```python
from build123d import *
from build123d.topology import SkipClean

# Parameters (mm, degrees)
SKETCH_1_R           = 112.5
SKETCH_1_R_2         = 90
EXTRUDE_1_DEPTH      = 3
EXTRUDE_START        = -60
EXTRUDE_2_DEPTH      = 60
SKETCH_5_R           = 2.75
CUT_EXTRUDE_1_DEPTH  = 10
EXTRUDE_3_DEPTH      = 5
EXTRUDE_3_DEPTH_BACK = 3
SKETCH_6_R           = 115.5
SKETCH_6_R_2         = 112.5
EXTRUDE_START_2      = 10
EXTRUDE_4_DEPTH      = 10


with BuildPart() as part:
    # Sketch 1 → Extrude 1 (new body)
    with BuildSketch(Plane.XY):
        Circle(SKETCH_1_R)
        Circle(SKETCH_1_R_2, mode=Mode.SUBTRACT)
    extrude(amount=EXTRUDE_1_DEPTH)

    # Sketch 4 → Extrude 2 (add)
    with BuildSketch(Plane.XY.offset(3).offset(EXTRUDE_START)):
        with BuildLine():
            Line((-25, 109.687054842), (-25, 112.76191733))
            ThreePointArc((-25, 112.76191733), (0, -115.5), (25, 112.76191733))
            Line((25, 112.76191733), (25, 109.687054842))
            ThreePointArc((25, 109.687054842), (0, -112.5), (-25, 109.687054842))
        make_face()
    extrude(amount=EXTRUDE_2_DEPTH)

    # Sketch 5 → Cut-Extrude 1 (cut)
    with BuildSketch(Plane.XY.offset(3)):
        with Locations((80, 60)):
            Circle(SKETCH_5_R)
        with Locations((92.803208809, 37.250025969)):
            Circle(SKETCH_5_R)
        with Locations((61.744923397, 78.661073186)):
            Circle(SKETCH_5_R)
        with Locations((61.744923397, -78.661073186)):
            Circle(SKETCH_5_R)
        with Locations((92.803208809, -37.250025969)):
            Circle(SKETCH_5_R)
        with Locations((80, -60)):
            Circle(SKETCH_5_R)
        with Locations((-80, -60)):
            Circle(SKETCH_5_R)
        with Locations((-92.803208809, -37.250025969)):
            Circle(SKETCH_5_R)
        with Locations((-61.744923397, -78.661073186)):
            Circle(SKETCH_5_R)
        with Locations((-61.744923397, 78.661073186)):
            Circle(SKETCH_5_R)
        with Locations((-92.803208809, 37.250025969)):
            Circle(SKETCH_5_R)
        with Locations((-80, 60)):
            Circle(SKETCH_5_R)
        with Locations((15, 105)):
            Circle(SKETCH_5_R)
        with Locations((-15, 105)):
            Circle(SKETCH_5_R)
    extrude(amount=-CUT_EXTRUDE_1_DEPTH, mode=Mode.SUBTRACT)

    # Sketch 6 → Extrude 3 (add, two sides: drawn at the far end of the back side and taken through both)
    with SkipClean():  # the faces are left unmerged after this step: merging them gives an invalid solid
        with BuildSketch(Plane(origin=(0, 0, 0), x_dir=(-1, 0, 0), z_dir=(0, 0, -1)).offset(-EXTRUDE_3_DEPTH_BACK)):
            with Locations(Location((0, 0, 0), (0, 0, 180))):
                Circle(SKETCH_6_R)
            with Locations(Location((0, 0, 0), (0, 0, 180))):
                Circle(SKETCH_6_R_2, mode=Mode.SUBTRACT)
        extrude(amount=EXTRUDE_3_DEPTH + EXTRUDE_3_DEPTH_BACK)

    # Sketch 7 → Extrude 4 (add)
    with SkipClean():  # the faces are left unmerged after this step: merging them gives an invalid solid
        with BuildSketch(Plane(origin=(0, 0, -57), x_dir=(-1, 0, 0), z_dir=(0, 0, -1)).offset(EXTRUDE_START_2)):
            with BuildLine():
                Line((-48.117044797, 105), (48.117044797, 105))
                ThreePointArc((48.117044797, 105), (36.763941575, 109.492751358), (25, 112.76191733))
                Line((25, 112.76191733), (25, 109.687054842))
                Line((25, 109.687054842), (-25, 109.687054842))
                Line((-25, 109.687054842), (-25, 112.76191733))
                ThreePointArc((-25, 112.76191733), (-36.763941575, 109.492751358), (-48.117044797, 105))
            make_face()
        extrude(amount=-EXTRUDE_4_DEPTH)


solid = part.part
```
Source: CAD feature listing. Evaluate the final solid. Frame: model axes, mm. A direction names the side the tool comes from. Give positions to 0.01 mm unless a question says otherwise; leave off trailing zeros. Order: outer loops, then holes, each group sorted by start corner. A loop starts at its lowest first (then second) coordinate and runs counter-clockwise, first axis right, second up. Notation, with made-up numbers: (36.5, -26.5) -> (77.5, -26.5) arc R37 ccw to (77.5, 9.5) -> close; hole circle Ø10 at (34, 36.25). An arc over 180 degrees is marked (long way). Use a Markdown table: item, result.
Q1. Section D-D (y = 8). Return the cut outline in (x, z), and give its area (3 significant figures).
A:
| item | result |
|---|---|
| outline | (-115.22, -57) -> (-112.22, -57) -> (-112.22, 0) -> (-89.64, 0) -> (-89.64, 3) -> (-115.22, 3) -> close; (89.64, 0) -> (112.22, 0) -> (112.22, -57) -> (115.22, -57) -> (115.22, 3) -> (89.64, 3) -> close |
| area | 496 mm^2 |
Q2. Access query for faces 1 (the face through (1, 107, -67)), 2 (the face through (-15.596, 102.315, 1.521)), 3 (the face through (0, 113, -5)). Directions: +Z, -Z, +X, -X, +Y, -Y. A direction counts if a zero-diameter tool reaches every point of the face in a straight line with its end or side. Return the directions, or none.
A:
| item | result |
|---|---|
| face 1 | -Z, +X, -X, +Y, -Y |
| face 2 | +Z |
| face 3 | -Z, +Y |
Q3. Section C-C (x = -80). Return the cut outline in (y, z), and give its area (3 significant figures).
A:
| item | result |
|---|---|
| outline | (-83.31, -57) -> (-79.1, -57) -> (-79.1, 0) -> (-62.75, 0) -> (-62.75, 3) -> (-83.31, 3) -> close; (-57.25, 0) -> (-41.23, 0) -> (-41.23, 3) -> (-57.25, 3) -> close; (41.23, 0) -> (57.25, 0) -> (57.25, 3) -> (41.23, 3) -> close; (62.75, 0) -> (79.1, 0) -> (79.1, -57) -> (83.31, -57) -> (83.31, 3) -> (62.75, 3) -> close |
| area | 700 mm^2 |
Q4. First-contact query: P1, Ø1, axis at y = 77.5, z = -35, coming from the -X side; P2, Ø7, axis at x = -61.74, y = 78.66, coming from the -Z side; P3, Ø4.5, axis at x = 92.8, y = 37.25, coming from the +Z side; P4, Ø5, axis at y = -46.5, z = -44, coming from the -X side. Flat tips, straight axial feed; report the tip coordinate or a pass-through.
A:
| item | result |
|---|---|
| P1 | x = -86.09 |
| P2 | z = 0 |
| P3 | through |
| P4 | x = -106.79 |
Q5. Material intervals for line 1 (Y direction, x = 0, z = 2.2); line 2 (Z direction, x = 66.5, y = 63); line 3 (Y direction, x = 38, z = -51), sorted ascending. Write a range as [from, to].
A:
| item | result |
|---|---|
| line 1 | [-115.5, -90], [90, 115.5] |
| line 2 | [0, 3] |
| line 3 | [-109.07, -105.89], [105.89, 109.07] |
Q6. Section B-B (y = 45.5). Return the cut outline in (x, z), and give its area (3 significant figures).
A:
| item | result |
|---|---|
| outline | (-106.16, -57) -> (-102.89, -57) -> (-102.89, 0) -> (-77.65, 0) -> (-77.65, 3) -> (-106.16, 3) -> close; (77.65, 0) -> (102.89, 0) -> (102.89, -57) -> (106.16, -57) -> (106.16, 3) -> (77.65, 3) -> close |
| area | 544 mm^2 |
Q7. Pull-direction query (Y, two-part tool) for faces 4 (the face through (1, 105, -62)), 5 (the face through (111, -21, -57)), 6 (the face through (63.01, 76.22, 1.52)); classes: +Y half, -Y half, draft (parallel to the pull), parting line (faces both ways), or undercut.
A:
| item | result |
|---|---|
| face 4 | -Y half |
| face 5 | draft |
| face 6 | undercut |
Q8. Section A-A (x = 0). Return the cut outline in (y, z), and give its area (3 significant figures).
A:
| item | result |
|---|---|
| outline | (-115.5, -57) -> (-112.5, -57) -> (-112.5, 0) -> (-90, 0) -> (-90, 3) -> (-115.5, 3) -> close; (90, 0) -> (112.5, 0) -> (112.5, -5) -> (115.5, -5) -> (115.5, 3) -> (90, 3) -> close; (105, -67) -> (109.69, -67) -> (109.69, -57) -> (105, -57) -> close |
| area | 386 mm^2 |
